The model under review builds one solid part; all positions refer to its coordinate system, in mm. A direction names the side the tool comes from. Coordinates: 2 decimals unless noted, no trailing zeros. Write each loop counter-clockwise with the first axis right and the second up, starting at its lowest first coordinate (ties: lowest second). Pieces come first, ordered by that corner, then holes. Notation, with made-up numbers: (48, 80.5) - (78, 80.5) arc R10 cw to (78, 98.5) - close; hole circle Ø8 at (5.25, 82.25). An arc over 180 degrees is marked (long way). Return JSON: item names as keys, results as strings. Group by question number.
(1) Draft analysis for pull direction Y (two halves, no side actions). For faces 1 (the face through (26, 18.75, -12)), 2 (the face through (-27.25, 17, -12)), 3 (the face through (20.5, -12.5, 1)), state which applies: released by +Y, released by -Y, zero draft, split by the parting line, or undercut.
(2) Tool access review of faces 4 (the face through (27.25, 17, -12)), 5 (the face through (0, 14, 1)), 6 (the face through (-26, -18.75, -12)): name each direction out of +Z, -Z, +X, -X, +Y, -Y from which nothing blocks a thin tool from reaching the whole face with its end or side.
(3) We need section D-D on y = -12.5. State the section outline as (x, z) points.
(4) To check wall thickness, follow L1, parallel to Y at x = 19, z = 1.25; L2, parallel to Z at x = -26, y = -3; L3, parallel to Y at x = -25, z = -13. State the ranges of each line that lie inside material, in increasing order. Write a range as from..to.
(5) We need section C-C on x = 9.5. State the section outline as (y, z) points, then the cut area to 3 significant figures.
(6) We need section B-B on y = 0. State the section outline as (x, z) points.
(7) We need section A-A on z = -11. State the section outline as (x, y) points, then the cut area to 3 significant figures.
(8) For pin 1 Ø1.2 at (y, z) = (17, -7.5) entering from +X; pin 2 Ø8 at (x, y) = (16.5, 3.5) entering from -Z; pin 3 Ø1.2 at (x, z) = (-25.5, -6.5) entering from +Y, all flat-tipped, find the tip position at first contact; note any pin that passes through.
```python
from build123d import *

# Parameters (mm, degrees)
SKETCH1_W           = 58
SKETCH1_H           = 40
BOSS_EXTRUDE2_DEPTH = 2
SKETCH2_R           = 7
CUT_EXTRUDE1_DEPTH  = 2
FILLET1_R           = 2
SKETCH4_R           = 2.5
CUT_EXTRUDE5_DEPTH  = 2
SKETCH6_R           = 2.5
BOSS_EXTRUDE3_DEPTH = 2
SKETCH7_W           = 2.5
SKETCH7_H           = 2.5
BOSS_EXTRUDE5_DEPTH = 30
SKETCH8_R           = 5
CUT_EXTRUDE6_DEPTH  = 66


with BuildPart() as part:
    # Sketch1 → Boss-Extrude2 (new body)
    with BuildSketch(Plane.XY):
        Rectangle(SKETCH1_W, SKETCH1_H)
    extrude(amount=BOSS_EXTRUDE2_DEPTH)

    # Sketch2 → Cut-Extrude1 (cut)
    with BuildSketch(Plane.XY.offset(2)):
        Circle(SKETCH2_R)
        with Locations((19, 0)):
            Circle(SKETCH2_R)
        with Locations((-19, 0)):
            Circle(SKETCH2_R)
        with BuildLine():
            Line((-19, 13.999747299), (19, 13.999747299))
            ThreePointArc((19, 13.999747299), (20.499747299, 12.5), (19, 11.000252701))
            Line((19, 11.000252701), (-19, 11.000252701))
            ThreePointArc((-19, 11.000252701), (-20.499747299, 12.5), (-19, 13.999747299))
        make_face()
        with BuildLine():
            Line((-19, -10.99999193), (19, -10.99999193))
            ThreePointArc((19, -10.99999193), (20.50000807, -12.5), (19, -14.00000807))
            Line((19, -14.00000807), (-19, -14.00000807))
            ThreePointArc((-19, -14.00000807), (-20.50000807, -12.5), (-19, -10.99999193))
        make_face()
    extrude(amount=-CUT_EXTRUDE1_DEPTH, mode=Mode.SUBTRACT)

    # Fillet1
    fillet1_edges = [part.edges().sort_by_distance(p)[0] for p in [
        (29, -20, 1),
        (-29, -20, 1),
        (-29, 20, 1),
        (29, 20, 1),
    ]]
    fillet(fillet1_edges, radius=FILLET1_R)

    # Sketch4 → Cut-Extrude5 (cut)
    with BuildSketch(Plane(origin=(0, 0, 0), x_dir=(-1, 0, 0), z_dir=(0, 0, -1))):
        with Locations((25.5, 12.5)):
            Circle(SKETCH4_R)
        with Locations(Location((25.5, -12.5, 0), (0, 0, 180))):
            Circle(SKETCH4_R)
        with Locations((-25.5, -12.5)):
            Circle(SKETCH4_R)
        with Locations(Location((-25.5, 12.5, 0), (0, 0, 180))):
            Circle(SKETCH4_R)
    extrude(amount=-CUT_EXTRUDE5_DEPTH, mode=Mode.SUBTRACT)

    # Sketch6 → Boss-Extrude3 (add)
    with BuildSketch(Plane(origin=(0, 0, 0), x_dir=(-1, 0, 0), z_dir=(0, 0, -1))):
        with Locations((25.5, 12.5)):
            Circle(SKETCH6_R)
        with Locations((25.5, -12.5)):
            Circle(SKETCH6_R)
        with Locations((-25.5, -12.5)):
            Circle(SKETCH6_R)
        with Locations((-25.5, 12.5)):
            Circle(SKETCH6_R)
    extrude(amount=-BOSS_EXTRUDE3_DEPTH)

    # Sketch7 → Boss-Extrude5 (add)
    with BuildSketch(Plane(origin=(0, 0, 0), x_dir=(-1, 0, 0), z_dir=(0, 0, -1))):
        with Locations((-26, 17.5)):
            Rectangle(SKETCH7_W, SKETCH7_H)
        with Locations((-26, -17.5)):
            Rectangle(SKETCH7_W, SKETCH7_H)
        with Locations((26, -17.5)):
            Rectangle(SKETCH7_W, SKETCH7_H)
        with Locations((26, 17.5)):
            Rectangle(SKETCH7_W, SKETCH7_H)
    extrude(amount=BOSS_EXTRUDE5_DEPTH)

    # Sketch8 → Cut-Extrude6 (cut)
    with BuildSketch(Plane.ZY.offset(27.25)):
        with Locations((-30, 17.5)):
            Circle(SKETCH8_R)
        with Locations((-30, -17.5)):
            Circle(SKETCH8_R)
    extrude(amount=-CUT_EXTRUDE6_DEPTH, mode=Mode.SUBTRACT)


solid = part.part
```
Ans:
{
 "1": {"face 1": "released by +Y", "face 2": "zero draft", "face 3": "undercut"},
 "2": {"face 4": "-Z, +X, +Y, -Y", "face 5": "+Z, -Z", "face 6": "-Z, +X, -X, -Y"},
 "3": {"outline": "(-29, 0) - (-20.5, 0) - (-20.5, 2) - (-29, 2) - close; (20.5, 0) - (29, 0) - (29, 2) - (20.5, 2) - close"},
 "4": {"L1": "-20..-14, -11..-7, 7..11, 14..20", "L2": "0..2", "L3": "-18.75..-16.25, 16.25..18.75"},
 "5": {"outline": "(-20, 0) - (-14, 0) - (-14, 2) - (-20, 2) - close; (-11, 0) - (11, 0) - (11, 2) - (-11, 2) - close; (14, 0) - (20, 0) - (20, 2) - (14, 2) - close", "area": "68.0 mm²"},
 "6": {"outline": "(-29, 0) - (-26, 0) - (-26, 2) - (-29, 2) - close; (-12, 0) - (-7, 0) - (-7, 2) - (-12, 2) - close; (7, 0) - (12, 0) - (12, 2) - (7, 2) - close; (26, 0) - (29, 0) - (29, 2) - (26, 2) - close"},
 "7": {"outline": "(-27.25, -18.75) - (-24.75, -18.75) - (-24.75, -16.25) - (-27.25, -16.25) - close; (-27.25, 16.25) - (-24.75, 16.25) - (-24.75, 18.75) - (-27.25, 18.75) - close; (24.75, -18.75) - (27.25, -18.75) - (27.25, -16.25) - (24.75, -16.25) - close; (24.75, 16.25) - (27.25, 16.25) - (27.25, 18.75) - (24.75, 18.75) - close", "area": "25.0 mm²"},
 "8": {"pin 1": "x = 27.25", "pin 2": "z = 0", "pin 3": "y = 18.75"}
}
